```python
from build123d import *

# Parameters (mm, degrees)
F0_R     = 14.2875
F1_DEPTH = 5.08


# Not quite as in the source:
# - a feature names something its author has since deleted; it is built from what else it names


with BuildPart() as f1:
    # F0 (on Top) → F1 (new body)
    with BuildSketch(Plane.XY):
        with BuildLine():
            ThreePointArc((0, 20), (5.8578643763, 5.8578643763), (20, 0))
            Line((20, 0), (37.5, 0))
            ThreePointArc((37.5, 0), (51.6421356237, 5.8578643763), (57.5, 20))
            Line((57.5, 20), (57.5, 158.715))
            ThreePointArc((57.5, 158.715), (28.75, 187.465), (0, 158.715))
            Line((0, 158.715), (0, 20))
        make_face()
        with Locations((28.75, 30)):
            Circle(F0_R, mode=Mode.SUBTRACT)
        with Locations((28.75, 158.715)):
            Circle(F0_R, mode=Mode.SUBTRACT)
    extrude(amount=F1_DEPTH)


solid = f1.part
```
Geometry: final body of the model. Coordinates: model frame, mm. Give positions to 0.01 mm unless a question says otherwise; leave off trailing zeros. Write each loop counter-clockwise with the first axis right and the second up, starting at its lowest first coordinate (ties: lowest second). Pieces come first, ordered by that corner, then holes.
1. Section query D-D, the plane x = 40.5. Return loops of the section in (y, z), then the cut area to 3 significant figures.
2. Line query: probe 1 along Y at (x, z) = (28.75, 1.55) (1 decimal); probe 2 along X at (y, z) = (158.5, 2.2); probe 3 along Y at (x, z) = (34.5, 3.5). Output: solid intervals per line, ascending.
3. Draft query along X for faces 1 (the cylindrical face through (25.653, 144.767, 2.504)), 2 (the flat face through (0, 90, 3)), 3 (the cylindrical face through (35.343, 17.325, 2.504)), 4 (the flat face through (29, 0, 3)). Return one class per face: released by +X, released by -X, zero draft, split by the parting line, or undercut.
4. Section query A-A, the plane z = 2.05. Count the separate pieces of the cut face and the enclosed holes in it, then the cut area to 3 significant figures.
5. Section query B-B, the plane y = 30. Return loops of the section in (x, z).
6. Pin query (flat end, axial travel): P1, Ø3, axis at x = 6, z = 2.5, coming from the +Y side; P2, Ø2, axis at x = 50, y = 66.5, coming from the -Z side; P3, Ø1, axis at x = 14.5, z = 2, coming from the +Y side. Return the tip coordinate at first contact, or that it passes through.
7. Section query C-C, the plane x = 28.75. Return loops of the section in (y, z) (1 decimal), then the cut area to 3 significant figures.
Computed:
1. outline: (0.23, 0) - (21.87, 0) - (21.87, 5.08) - (0.23, 5.08) - close; (38.13, 0) - (150.59, 0) - (150.59, 5.08) - (38.13, 5.08) - close; (166.84, 0) - (184.95, 0) - (184.95, 5.08) - (166.84, 5.08) - close
1. area: 773 mm2
2. probe 1: y = 0 to 15.7, 44.3 to 144.4, 173 to 187.5
2. probe 2: x = 0 to 14.46, 43.04 to 57.5
2. probe 3: y = 0 to 16.92, 43.08 to 145.64, 171.79 to 186.88
3. face 1: undercut
3. face 2: released by -X
3. face 3: undercut
3. face 4: zero draft
4. separate pieces: 1
4. enclosed holes: 2
4. area: 8,970 mm2
5. outline: (0, 0) - (14.46, 0) - (14.46, 5.08) - (0, 5.08) - close; (43.04, 0) - (57.5, 0) - (57.5, 5.08) - (43.04, 5.08) - close
6. P1: stops at y = 178.08
6. P2: stops at z = 0
6. P3: stops at y = 183.96
7. outline: (0, 0) - (15.7, 0) - (15.7, 5.1) - (0, 5.1) - close; (44.3, 0) - (144.4, 0) - (144.4, 5.1) - (44.3, 5.1) - close; (173, 0) - (187.5, 0) - (187.5, 5.1) - (173, 5.1) - close
7. area: 662 mm2
